```python
from build123d import *

# Parameters (mm, degrees)
F0_R     = 1.5
F1_DEPTH = 2.5


# Not quite as in the source:
# - ends of sketch curves that miss each other by under 0.0002 mm in the source are joined


with BuildPart() as f1:
    # F0 (on Top) → F1 (new body)
    with BuildSketch(Plane.XY):
        with BuildLine():
            ThreePointArc((148.553042, 14.928769), (146.7956826871, 19.1714096871), (142.553042, 20.928769))
            Line((142.553042, 20.928769), (61.546959, 20.928769))
            ThreePointArc((61.546959, 20.928769), (57.3043183129, 22.6861283129), (55.546959, 26.928769))
            Line((55.546959, 26.928769), (55.546959, 35.928769))
            ThreePointArc((55.546959, 35.928769), (54.6682793436, 38.0500893436), (52.546959, 38.928769))
            Line((52.546959, 38.928769), (-8.453041, 38.928769))
            Line((-8.453041, 38.928769), (-89.559124, 18.860903))
            ThreePointArc((-89.559124, 18.860903), (-96.6607350116, 19.7413862614), (-101.3556837465, 25.1419037277))
            ThreePointArc((-101.3556837465, 25.1419037277), (-106.6281165379, 28.3955877128), (-111.0175785103, 24.0232160611))
            ThreePointArc((-111.0175785103, 24.0232160611), (-112.2824719314, 21.9176106757), (-114.6963029885, 21.462694048))
            ThreePointArc((-114.6963029885, 21.462694048), (-118.4956024313, 22.0698924501), (-122.3430789933, 22.0869199077))
            ThreePointArc((-122.3430789933, 22.0869199077), (-124.651171475, 22.9272997317), (-125.557821603, 25.2101739826))
            ThreePointArc((-125.557821603, 25.2101739826), (-128.4655562478, 29.9721606196), (-133.972746844, 29.0764548336))
            Line((-133.972746844, 29.0764548336), (-145.972747, 17.826455))
            ThreePointArc((-145.972747, 17.826455), (-147.027366593, 16.4104523305), (-147.524076258, 14.7161780279))
            Line((-147.524076258, 14.7161780279), (-148.524076, 5.466178))
            ThreePointArc((-148.524076, 5.466178), (-148.0067044123, 2.6561312792), (-146.0349377658, 0.5882404096))
            ThreePointArc((-146.0349377658, 0.5882404096), (-144.929137249, -0.5106558369), (-144.524076, -2.016077))
            Line((-144.524076, -2.016077), (-144.524076, -32.126386))
            ThreePointArc((-144.524076, -32.126386), (-144.929137249, -33.6318071631), (-146.0349379189, -34.7307031419))
            ThreePointArc((-146.0349379189, -34.7307031419), (-148.0285132018, -36.8418479978), (-148.5127305604, -39.7048550716))
            Line((-148.5127305604, -39.7048550716), (-147.333918, -48.932011))
            ThreePointArc((-147.333918, -48.932011), (-146.8569609625, -50.4905877681), (-145.8877919349, -51.801068932))
            Line((-145.8877919349, -51.801068932), (-134.012517, -63.181221))
            ThreePointArc((-134.012517, -63.181221), (-128.2758744449, -64.0225805122), (-125.6012880056, -58.8783080008))
            ThreePointArc((-125.6012880056, -58.8783080008), (-124.8721529677, -56.4691107751), (-122.564742997, -55.4632638637))
            ThreePointArc((-122.564742997, -55.4632638637), (-118.5664827026, -55.3440377294), (-114.6018211423, -54.8132282387))
            ThreePointArc((-114.6018211423, -54.8132282387), (-112.1618303627, -55.4315323166), (-111.051616739, -57.6905760176))
            ThreePointArc((-111.051616739, -57.6905760176), (-106.8640436675, -62.5050200787), (-101.3556836703, -59.2843667555))
            ThreePointArc((-101.3556836703, -59.2843667555), (-96.6607350116, -53.8838492614), (-89.5591238689, -53.0033654703))
            Line((-89.5591238689, -53.0033654703), (-8.453041, -73.071231))
            Line((-8.453041, -73.071231), (52.546959, -73.071231))
            ThreePointArc((52.546959, -73.071231), (54.6682793436, -72.1925513436), (55.546959, -70.071231))
            Line((55.546959, -70.071231), (55.546959, -61.071231))
            ThreePointArc((55.546959, -61.071231), (57.3043183129, -56.8285903129), (61.546959, -55.071231))
            Line((61.546959, -55.071231), (142.553042, -55.071231))
            ThreePointArc((142.553042, -55.071231), (146.7956826871, -53.3138716871), (148.553042, -49.071231))
            Line((148.553042, -49.071231), (148.553042, -39.867925))
            ThreePointArc((148.553042, -39.867925), (148.4525408985, -39.0979210147), (148.1577712418, -38.3795078619))
            Line((148.1577712418, -38.3795078619), (144.750677, -32.417093))
            ThreePointArc((144.750677, -32.417093), (144.6032924632, -32.057886663), (144.553042, -31.672885))
            Line((144.553042, -31.672885), (144.553042, -2.469578))
            ThreePointArc((144.553042, -2.469578), (144.6032924632, -2.084576337), (144.7506770407, -1.7253700232))
            Line((144.7506770407, -1.7253700232), (148.157771, 4.237045))
            ThreePointArc((148.157771, 4.237045), (148.4525408985, 4.9554580147), (148.553042, 5.725462))
            Line((148.553042, 5.725462), (148.553042, 14.928769))
        make_face()
        with Locations((-130.553041, -59.571231)):
            Circle(F0_R, mode=Mode.SUBTRACT)
        with Locations((-106.053041, -57.571231)):
            Circle(F0_R, mode=Mode.SUBTRACT)
        with Locations((-52.553041, -31.571231)):
            Circle(F0_R, mode=Mode.SUBTRACT)
        with Locations((116.346959, -41.071231)):
            Circle(F0_R, mode=Mode.SUBTRACT)
        with Locations((-106.053041, 23.428769)):
            Circle(F0_R, mode=Mode.SUBTRACT)
        with Locations((-130.553041, 25.428769)):
            Circle(F0_R, mode=Mode.SUBTRACT)
        with Locations((-48.053041, 18.428769)):
            Circle(F0_R, mode=Mode.SUBTRACT)
        with Locations((55.546959, -17.071231)):
            Circle(F0_R, mode=Mode.SUBTRACT)
        with Locations((116.346959, -17.071231)):
            Circle(F0_R, mode=Mode.SUBTRACT)
        with Locations((116.346959, 6.928769)):
            Circle(F0_R, mode=Mode.SUBTRACT)
    extrude(amount=-F1_DEPTH)


solid = f1.part
```
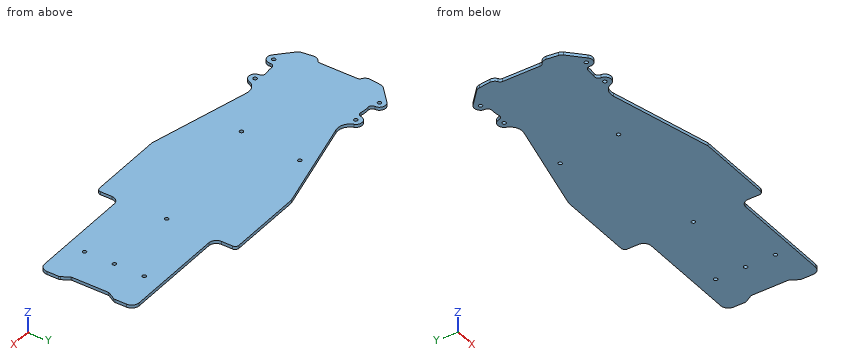
Verification items for the finished model (mm, model axes). Round coordinates to 2 decimals unless told otherwise and drop trailing zeros. Write each loop counter-clockwise with the first axis right and the second up, starting at its lowest first coordinate (ties: lowest second). Pieces come first, ordered by that corner, then holes.
1. Section check A-A on y = -27.5. Enter the section's corners in (x, z), plus the area to 3 significant figures.
2. Gauge pin test, flat ends, axial feed: P1, Ø1.2, axis at y = 33, z = -2, coming from the +X side; P2, Ø1, axis at y = -23.5, z = -0.5, coming from the -X side; P3, Ø1.5, axis at y = 18, z = -0.5, coming from the +X side. Record the tip position at first contact, or that the pin passes through.
3. Scan lines: L1, parallel to X at y = -17.5, z = -1.4; L2, parallel to X at y = -30, z = -0.4; L3, parallel to Y at x = 108.5, z = -1.05. Record each from-to range of solid material in increasing order.
4. Section check C-C on z = -1.95. State how many separate pieces and enclosed holes the cut face has, plus the area to 3 significant figures.
5. Section check B-B on x = 69. Enter the section's corners in (y, z), plus the area to 3 significant figures.
Answer:
1. outline: (-144.52, -2.5) - (144.55, -2.5) - (144.55, 0) - (-144.52, 0) - close
1. area: 723 mm2
2. P1: stops at x = 55.55
2. P2: stops at x = -144.52
2. P3: stops at x = 148.09
3. L1: x = -144.52 to 54.11, 56.98 to 114.91, 117.78 to 144.55
3. L2: x = -144.52 to 144.55
3. L3: y = -55.07 to 20.93
4. separate pieces: 1
4. enclosed holes: 10
4. area: 26,100 mm2
5. outline: (-55.07, -2.5) - (20.93, -2.5) - (20.93, 0) - (-55.07, 0) - close
5. area: 190 mm2
